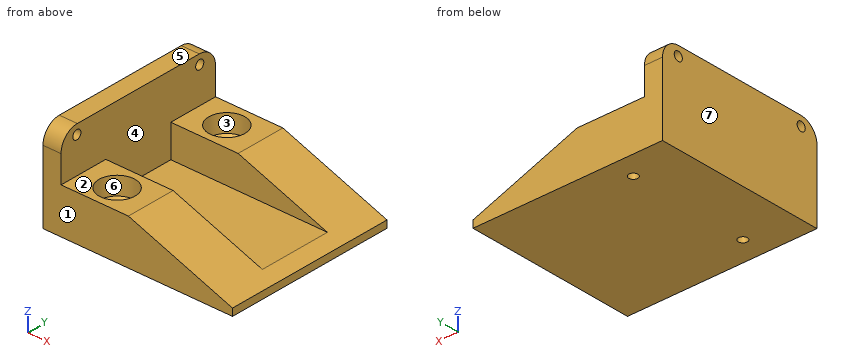
from build123d import *

# Parameters (mm, degrees)
F1_DEPTH  = 47.5
F2_W      = 86.76
F2_H      = 40
F3_DEPTH  = 18
F4_R      = 10
F5_R      = 2.5
F6_DEPTH  = 10
F8_D      = 20
F8_DEPTH  = 10
F8_TIP    = 6.0086061903
F9_R      = 2.5
F10_DEPTH = 25
F12_D     = 20
F12_DEPTH = 10
F12_TIP   = 6.0086061903
F13_R     = 2.5
F14_DEPTH = 25


with BuildPart() as f1:
    # F0 (on Front) → F1 (new body, symmetric)
    with BuildSketch(Plane.XZ):
        Polygon((-37.3029741915, -7.6123222187), (-47.3029741915, -7.6123222187), (-47.3029741915, -57.6123222187), (-37.3029741915, -57.6123222187), (-37.3029741915, -32.6123222187), align=None)
        Polygon((0, -32.6123222187), (-37.3029741915, -32.6123222187), (-37.3029741915, -57.6123222187), (57.6970258085, -57.6123222187), (57.6970258085, -53.6123222187), align=None)
    extrude(amount=F1_DEPTH, both=True)

    # F2 (on face) → F3 (cut)
    with BuildSketch(Plane.XY.offset(-32.6123222187)):
        with Locations((6.0770258085, 0)):
            Rectangle(F2_W, F2_H)
    extrude(amount=-F3_DEPTH, mode=Mode.SUBTRACT)

    # F4
    f4_edges = [f1.edges().sort_by_distance(p)[0] for p in [
        (-42.302974, -47.5, -7.612322),
        (-42.302974, 47.5, -7.612322),
    ]]
    fillet(f4_edges, radius=F4_R)

    # F5 (on face) → F6 (cut, through all)
    with BuildSketch(Plane.YZ.offset(-37.3029741915)):
        with Locations((-37.7820432186, -12.8668630496)):
            Circle(F5_R)
        with Locations((37.7820432186, -12.8668630496)):
            Circle(F5_R)
    extrude(amount=-F6_DEPTH, mode=Mode.SUBTRACT)

    # F8
    with Locations(Plane.XY.offset(-32.6123222187)):
        with Locations((-18.6514870957, -33.75)):
            Hole(F8_D / 2, depth=F8_DEPTH)
            with Locations((0, 0, -(F8_DEPTH + F8_TIP / 2))):  # 118° drill point
                Cone(0, F8_D / 2, F8_TIP, mode=Mode.SUBTRACT)

    # F9 (on face) → F10 (cut)
    with BuildSketch(Plane.XY.offset(-32.6123222187)):
        with Locations((-18.6514870957, -33.75)):
            Circle(F9_R)
    extrude(amount=-F10_DEPTH, mode=Mode.SUBTRACT)

    # F12
    with Locations(Plane.XY.offset(-32.6123222187)):
        with Locations((-18.6514870957, 33.75)):
            Hole(F12_D / 2, depth=F12_DEPTH)
            with Locations((0, 0, -(F12_DEPTH + F12_TIP / 2))):  # 118° drill point
                Cone(0, F12_D / 2, F12_TIP, mode=Mode.SUBTRACT)

    # F13 (on face) → F14 (cut)
    with BuildSketch(Plane.XY.offset(-32.6123222187)):
        with Locations((-19.2217435688, 34.2478714883)):
            Circle(F13_R)
    extrude(amount=-F14_DEPTH, mode=Mode.SUBTRACT)


solid = f1.part
Design review of the part built by this model. Coordinates are the model's own, in mm. Face numbers are marked on the shaded views. A direction names the side the tool comes from. Coordinates: 2 decimals unless noted, no trailing zeros. Order: outer loops, then holes, each group sorted by start corner. A loop starts at its lowest first (then second) coordinate and runs counter-clockwise, first axis right, second up. Notation, with made-up numbers: (-38, 26.25) - (-21, 26.25) arc R24 ccw to (-21, 46.25) - close; hole circle Ø7 at (-15.5, -24.75). An arc over 180 degrees is marked (long way). Put each result on its own line as item: value.
1) Tool access review of the marked faces 1, 2, 3 and 4: name each direction out of +Z, -Z, +X, -X, +Y, -Y from which nothing blocks a thin tool from reaching the whole face with its end or side.
Response values:
face 1: +Z, -Z, +X, -X, -Y
face 2: +Z, +X, +Y, -Y
face 3: +Z
face 4: +Z, +X
2) Take a section at B-B, the plane z = -44.5. Give the boundary of the cut face in (x, y), and give its area (3 significant figures).
Response values:
outline: (-47.3, -47.5) - (32.66, -47.5) - (32.66, -20) - (-37.3, -20) - (-37.3, 20) - (32.66, 20) - (32.66, 47.5) - (-47.3, 47.5) - close; hole circle Ø13.72 at (-18.65, -33.75); hole circle Ø13.72 at (-18.65, 33.75)
area: 4,500 mm²
3) Wall thickness on L1, parallel to X at y = -24.5, z = -26; L2, parallel to Z at x = -36.5, y = -26.5; L3, parallel to Z at x = -31, y = -9.5: over which ranges is each line inside the solid? List them lowest first. Write a range as from..to.
Response values:
L1: x = -47.3..-37.3
L2: z = -57.61..-32.61
L3: z = -57.61..-50.61
4) Insertion check: P1, Ø14, axis at x = -17, y = 31.5, coming from the +Z side; P2, Ø12, axis at x = -18.65, y = 33.75, coming from the +Z side; P3, Ø1.5, axis at x = 38, y = 27, coming from the +Z side; P4, Ø4, axis at x = -19.22, y = 34.25, coming from the -Z side. Each pin has a flat end and moves straight along its axis. Give the tip position at first contact, or say it passes through.
Response values:
P1: stops at z = -42.74
P2: stops at z = -45.01
P3: stops at z = -46.17
P4: passes through
5) Take a section at C-C, the plane x = -30. Give the boundary of the cut face in (y, z), and give its area (4 significant figures).
Response values:
outline: (-47.5, -57.61) - (47.5, -57.61) - (47.5, -32.61) - (20, -32.61) - (20, -50.61) - (-20, -50.61) - (-20, -32.61) - (-47.5, -32.61) - close
area: 1,655 mm²
6) Take a section at D-D, the plane y = -1. Give the boundary of the cut face in (x, z), and give its area (3 significant figures).
Response values:
outline: (-47.3, -57.61) - (57.7, -57.61) - (57.7, -53.61) - (49.45, -50.61) - (-37.3, -50.61) - (-37.3, -7.61) - (-47.3, -7.61) - close
area: 1,150 mm²
7) The part is to be moulded in two halves that separate along X. For the marked faces 5, 6 and 7, say which applies: released by +X, released by -X, zero draft, split by the parting line, or undercut.
Response values:
face 5: zero draft
face 6: undercut
face 7: released by -X
8) Take a section at A-A, the plane y = -33.75. Give the boundary of the cut face in (x, z).
Response values:
outline: (-47.3, -57.61) - (-21.15, -57.61) - (-21.15, -47.12) - (-28.65, -42.61) - (-28.65, -32.61) - (-37.3, -32.61) - (-37.3, -7.61) - (-47.3, -7.61) - close; (-16.15, -57.61) - (57.7, -57.61) - (57.7, -53.61) - (0, -32.61) - (-8.65, -32.61) - (-8.65, -42.61) - (-16.15, -47.12) - close
